Part model, mm, in its own coordinate system. A direction names the side the tool comes from. Round coordinates to 2 decimals unless told otherwise and drop trailing zeros. Loops run counter-clockwise (first coordinate to the right, second up) from the corner with the lowest first, then second, coordinate; pieces in that order, holes last. Notation, with made-up numbers: M -37.5,62 L 3.5,62 A10 ccw 3.5,69 Z; hole C 53,61 d8. An arc over 180 degrees is marked long. Write each question's results on one line, items separated by ' | '.
from build123d import *

# Parameters (mm, degrees)
BOSS_EXTRUDE2_DEPTH = 3
SKETCH2_W           = 12.5
SKETCH2_H           = 3
CUT_EXTRUDE1_DEPTH  = 3


with BuildPart() as part:
    # Sketch1 → Boss-Extrude2 (new body)
    with BuildSketch(Plane(origin=(0, 0, 0), x_dir=(0, 0, -1), z_dir=(1, 0, 0))):
        with BuildLine():
            Line((125, 0), (125, 1.5))
            ThreePointArc((125, 1.5), (111.75, 13.25), (100, 0))
            ThreePointArc((100, 0), (87.904372108, -47.674116292), (54.543572715, -83.81526517))
            add(Edge.make_bspline(
                [(54.543572715, -83.81526517), (44.434436781, -92.608940988), (31.581333534, -102.945692353), (30, -118.5)],
                knots=[0, 0, 0, 0, 1, 1, 1, 1], degree=3))
            Line((30, -118.5), (30, -121.5))
            ThreePointArc((30, -121.5), (42.5, -134), (55, -121.5))
            Line((55, -121.5), (55, -118.5))
            add(Edge.make_bspline(
                [(55, -118.5), (57.384287812, -110.868607185), (64.548856078, -107.860641761), (72.347282186, -101.935620665)],
                knots=[0, 0, 0, 0, 1, 1, 1, 1], degree=3))
            ThreePointArc((72.347282186, -101.935620665), (111.059466668, -57.365450084), (125, 0))
        make_face()
    extrude(amount=BOSS_EXTRUDE2_DEPTH)

    # Sketch2 → Cut-Extrude1 (cut)
    with BuildSketch(Plane(origin=(3, 0, 0), x_dir=(0, 0, -1), z_dir=(1, 0, 0))):
        with Locations((118.75, 0.8091646)):
            Rectangle(SKETCH2_W, SKETCH2_H)
        with Locations((48.75, -120)):
            Rectangle(SKETCH2_W, SKETCH2_H)
    extrude(amount=-CUT_EXTRUDE1_DEPTH, mode=Mode.SUBTRACT)


solid = part.part
Item 1: Band-saw the part on A-A on y = -48. Give the cut face in (x, z), and give its area (3 significant figures).
Filled sheet:
outline: M 0,-115.42 L 3,-115.42 L 3,-87.73 L 0,-87.73 Z | area: 83.1 mm^2
Item 2: Band-saw the part on B-B on z = -77. Give the cut face in (x, y).
Filled sheet:
outline: M 0,-98.47 L 3,-98.47 L 3,-63.8 L 0,-63.8 Z
Item 3: Wall check: L1, parallel to Z at x = 0.6, y = -54.5; L2, parallel to Y at x = 1.9, z = -114; L3, parallel to Y at x = 2.65, z = -51. Give the ranges that are in metal, low to high.
Filled sheet:
L1: -112.49 to -83.84 | L2: -51.27 to -0.69, 2.31 to 13.18 | L3: -130.67 to -121.5, -118.5 to -86.89
Item 4: Two-plate mould, pull along Y, no slides. Class faces 3 (the flat face through (3, -65, -84)), 4 (the flat face through (2, -118.5, -49)), 5 (the cylindrical face through (1.479, -58.407, -110.515)): +Y half, -Y half, draft (parallel to the pull), parting line (faces both ways), or undercut.
Filled sheet:
face 3: draft | face 4: undercut | face 5: -Y half
Item 5: Drop flat-ended pins along their axis: P1, Ø1.5, axis at x = 1.5, z = -47, coming from the +Y side; P2, Ø0.9, axis at x = 1.5, y = -119.5, coming from the -Z side; P3, Ø0.9, axis at x = 2, z = -47, coming from the -Y side. Give the stop position or say it passes through.
Filled sheet:
P1: y = -89.77 | P2: z = -42.5 | P3: y = -133.33
Item 6: Which spindle directions (+Z, -Z, +X, -X, +Y, -Y) get a long thin tool onto all of the face, cutting with end or side? Do faces 1 (the cylindrical face through (1.479, -133.997, -42.225)), 2 (the flat face through (2, -0.691, -119)). Say none if no direction does.
Filled sheet:
face 1: +X, -X, -Y | face 2: -Z, +X, -X
